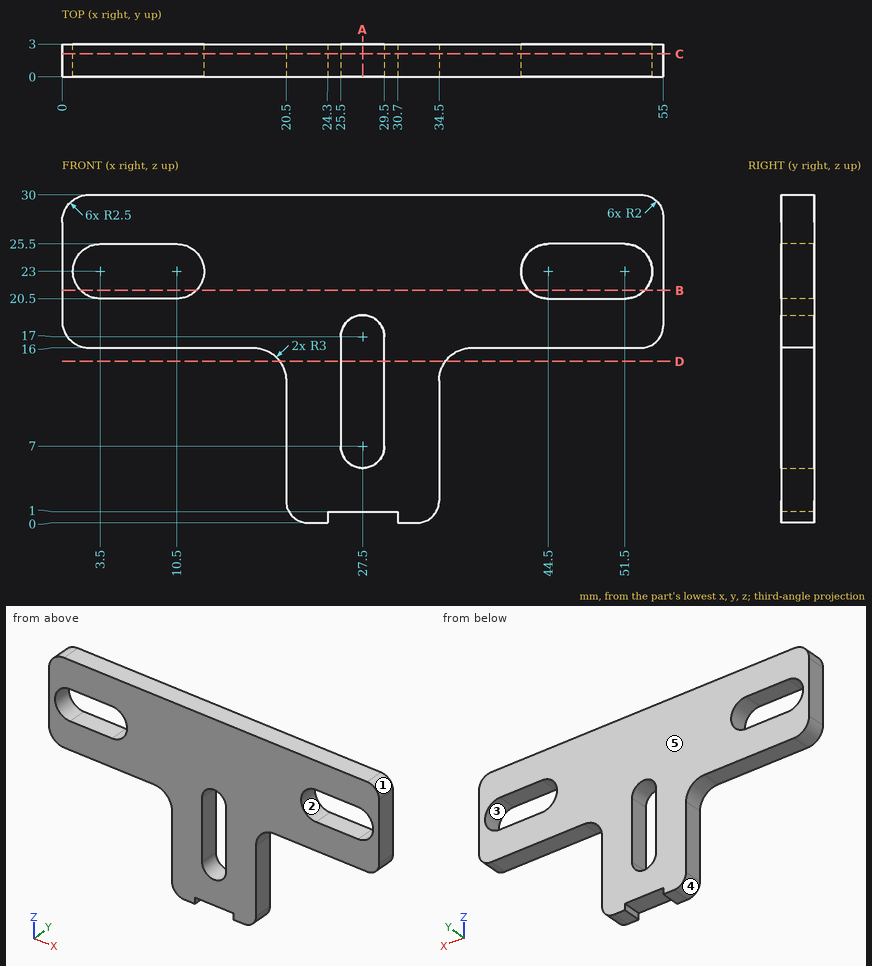
Here's the drawing with two shaded views (mm, measured from the low corner). I have some questions. A direction names the side the tool comes from. Give positions to 0.01 mm unless a question says otherwise; leave off trailing zeros. Loops run counter-clockwise (first coordinate to the right, second up) from the corner with the lowest first, then second, coordinate; pieces in that order, holes last. Notation, with made-up numbers: M 29,48.5 L 52,48.5 A11 cw 52,65.5 Z; hole C 12.25,84 d7. An arc over 180 degrees is marked long. One line per item, written item: value. Start each with the question number.
1) If we section it at D-D, the plane z = 14.75: Write out the boundary of the cut face in (x, y).
2) If we section it at C-C, the plane y = 2.1: Give the number of separate pieces and of enclosed holes in the cut face, and give its area (3 significant figures).
3) On a 3-axis mill with a long thin cutter (end or side, diameter ignored), from which of +Z, -Z, +X, -X, +Y, -Y can I reach the whole of each face in a straight line? I mean the marked faces 1 and 2. Say none if no direction works.
4) If I drill on line 1 (X direction, y = 0.25, z = 22.75); line 2 (Z direction, x = 4, y = 1.8); line 3 (X direction, y = 1.55, z = 8.75), over which ranges is the centre line in solid material (lowest first)? Write a range as [from, to].
5) If we section it at A-A, the plane x = 27.5: Write out the boundary of the cut face in (y, z).
6) I'm going to push flat-ended pins straight in: pin 1 (1.1 mm diameter, centred on y = 2, z = 0.5, fed in from +X); pin 2 (1.5 mm diameter, centred on y = 1, z = 12.5, fed in from +X); pin 3 (1.5 mm diameter, centred on x = 46.5, y = 1, fed in from -Z). Where does each tip first touch, or does it pass through?
7) Thinking about a two-plate mould opening in Z: for the marked faces 3, 4 and 5, which applies, +Z half, -Z half, draft (parallel to the pull), parting line (faces both ways), or undercut?
8) If we section it at B-B, the plane z = 21.25: Write out the boundary of the cut face in (x, y).
Completed:
1. outline: M 19.94,0 L 25.5,0 L 25.5,3 L 19.94,3 Z; M 29.5,0 L 35.06,0 L 35.06,3 L 29.5,3 Z
2. separate pieces: 1
2. enclosed holes: 3
2. area: 824 mm^2
3. face 1: +Z, +X, +Y, -Y
3. face 2: +Y, -Y
4. line 1: x = [0, 1.01], [12.99, 42.01], [53.99, 55]
4. line 2: z = [16, 20.5], [25.5, 30]
4. line 3: x = [20.5, 25.5], [29.5, 34.5]
5. outline: M 0,1 L 3,1 L 3,5 L 0,5 Z; M 0,19 L 3,19 L 3,30 L 0,30 Z
6. pin 1: stops at x = 34.26
6. pin 2: stops at x = 34.51
6. pin 3: stops at z = 16
7. face 3: undercut
7. face 4: -Z half
7. face 5: draft
8. outline: M 0,0 L 1.71,0 L 1.71,3 L 0,3 Z; M 12.29,0 L 42.71,0 L 42.71,3 L 12.29,3 Z; M 53.29,0 L 55,0 L 55,3 L 53.29,3 Z
